from build123d import *

# Parameters (mm, degrees)
BOSS_EXTRUDE1_DEPTH      = 32
CUT_EXTRUDE5_DEPTH       = 3.999999672
LPATTERN1_COUNT          = 5
LPATTERN1_PITCH          = 7
LPATTERN2_COUNT          = 5
LPATTERN2_PITCH          = 6
SKETCH12_W               = 8
SKETCH12_H               = 4
CUT_EXTRUDE7_DEPTH       = 12
CUT_EXTRUDE8_DEPTH       = 17
CUT_EXTRUDE8_DEPTH_BACK  = 4
SKETCH11_W               = 8
SKETCH11_H               = 31.059426665
CUT_EXTRUDE10_DEPTH      = 17
CUT_EXTRUDE10_DEPTH_BACK = 4
SKETCH13_W               = 10.75
SKETCH13_H               = 28.869342983
SKETCH13_W_2             = 7.056880225
SKETCH13_H_2             = 29.936318605
F_4_0MM_DOWEL_HOLE1_D    = 4


with BuildPart() as part:
    # Sketch1 → Boss-Extrude1 (new, symmetric)
    with BuildSketch(Plane.XY):
        Polygon((-23.75, 31.999999672), (23.75, 31.999999672), (23.75, 8), (29, 8), (29, 4), (21, 4), (21, 18), (18.25, 18), (18.25, 28), (-18.25, 28), (-18.25, 18), (-21, 18), (-21, 4), (-29, 4), (-29, 8), (-23.75, 8), align=None)
    extrude(amount=BOSS_EXTRUDE1_DEPTH, both=True)

    # Sketch8 → Cut-Extrude5 (cut)
    with BuildSketch(Plane(origin=(0, 31.999999672, 0), x_dir=(1, 0, 0), z_dir=(0, 1, 0))):
        with BuildLine():
            Line((11.25, -2.8), (-11.25, -2.8))
            ThreePointArc((-11.25, -2.8), (-11.957106781, -2.507106781), (-12.25, -1.8))
            Line((-12.25, -1.8), (-12.25, -1))
            ThreePointArc((-12.25, -1), (-11.957106781, -0.292893219), (-11.25, 0))
            Line((-11.25, 0), (11.25, 0))
            ThreePointArc((11.25, 0), (11.957106781, -0.292893219), (12.25, -1))
            Line((12.25, -1), (12.25, -1.8))
            ThreePointArc((12.25, -1.8), (11.957106781, -2.507106781), (11.25, -2.8))
        make_face()
    cut_extrude5 = extrude(amount=-CUT_EXTRUDE5_DEPTH, mode=Mode.SUBTRACT)

    # LPattern1: Cut-Extrude5 ×5
    with Locations(*[(0, 0, -i * LPATTERN1_PITCH) for i in range(1, LPATTERN1_COUNT)]):
        add(cut_extrude5, mode=Mode.SUBTRACT)

    # LPattern2: Cut-Extrude5 ×5
    with Locations(*[(0, 0, i * LPATTERN2_PITCH) for i in range(1, LPATTERN2_COUNT)]):
        add(cut_extrude5, mode=Mode.SUBTRACT)

    # Sketch12 → Cut-Extrude7 (cut)
    with BuildSketch(Plane(origin=(0, 0, -32), x_dir=(-1, 0, 0), z_dir=(0, 0, -1))):
        with Locations((25, 6)):
            Rectangle(SKETCH12_W, SKETCH12_H)
        with Locations((-25, 6)):
            Rectangle(SKETCH12_W, SKETCH12_H)
    cut_extrude7 = extrude(amount=-CUT_EXTRUDE7_DEPTH, mode=Mode.SUBTRACT)

    # Mirror1: Cut-Extrude7 across plane
    add(cut_extrude7.mirror(Plane.XY), mode=Mode.SUBTRACT)

    # Sketch11 → Cut-Extrude8 (cut, two sides: drawn at the far end of the back side and taken through both)
    with BuildSketch(Plane(origin=(0, 0, -15), x_dir=(-1, 0, 0), z_dir=(0, 0, -1)).offset(-CUT_EXTRUDE8_DEPTH_BACK)):
        with Locations((25, 23.529713333)):
            Rectangle(SKETCH11_W, SKETCH11_H)
        with Locations((-25, 23.529713333)):
            Rectangle(SKETCH11_W, SKETCH11_H)
    extrude(amount=CUT_EXTRUDE8_DEPTH + CUT_EXTRUDE8_DEPTH_BACK, mode=Mode.SUBTRACT)

    # Sketch13 → Cut-Extrude10 (cut, two sides: drawn at the far end of the back side and taken through both)
    with BuildSketch(Plane.XY.offset(15).offset(-CUT_EXTRUDE10_DEPTH_BACK)):
        with Locations((26.375, 22.434671492)):
            Rectangle(SKETCH13_W, SKETCH13_H)
        with Locations((-24.528440113, 22.968159303)):
            Rectangle(SKETCH13_W_2, SKETCH13_H_2)
    extrude(amount=CUT_EXTRUDE10_DEPTH + CUT_EXTRUDE10_DEPTH_BACK, mode=Mode.SUBTRACT)

    # Ø4.0mm Dowel Hole1 (through all)
    with Locations(Plane(origin=(0, 8, 0), x_dir=(1, 0, 0), z_dir=(0, 1, 0))):
        with Locations((25, -15), (25, 15), (-25, 15), (-25, -15)):
            Hole(F_4_0MM_DOWEL_HOLE1_D / 2)


solid = part.part
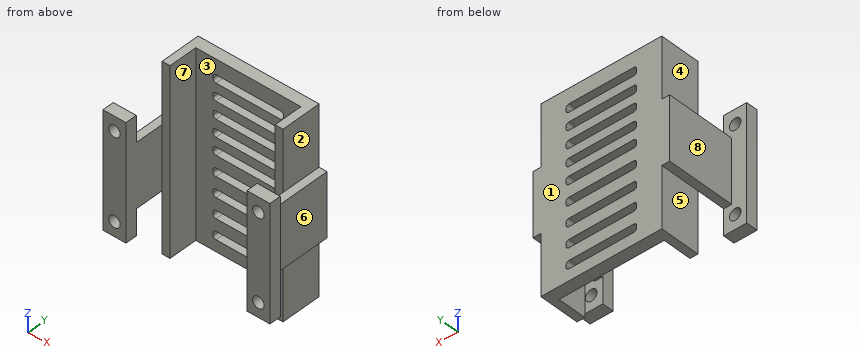
Build history of the part. All positions in model axes, mm. Face numbers are marked on the shaded views. A direction names the side the tool comes from. Coordinates: 2 decimals unless noted, no trailing zeros. Order: outer loops, then holes, each group sorted by start corner. A loop starts at its lowest first (then second) coordinate and runs counter-clockwise, first axis right, second up. Notation, with made-up numbers: (55.5, 4) - (63.5, 4) arc R22 cw to (63.5, 21) - close; hole circle Ø3 at (-23, 80.5). An arc over 180 degrees is marked (long way). Write item = value, one per line. Start each with the question number.
1) Saw through at C-C on y = 10.25. Write the cut outline in (x, z), then the cut area to 3 significant figures.
2) 3-axis set-ups, long thin cutter, end or side, ignore diameter. For the marked faces 4, 5, 6, 7 and 8: which of +Z, -Z, +X, -X, +Y, -Y reach the whole face in a straight line?
3) Wall check: line 1 along X through (y, z) = (6.65, -15); line 2 along Z through (x, y) = (-25, 6.05); line 3 along X through (y, z) = (22.5, -23.5). Give the ranges that are in metal, low to high. Write a range as from..to.
4) Two-plate mould, pull along X, no slides. Class the marked faces 1, 2 and 3: pulls with the +X half, pulls with the -X half, needs draft (parallel to the pull), parting line crosses it, or undercut.
5) Saw through at A-A on z = -15. Write the cut outline in (x, y).
6) Saw through at B-B on x = 25. Write the cut outline in (y, z), then the cut area to 3 significant figures.
7) Saw through at D-D on z = -8. Write the cut outline in (x, y), then the cut area to 3 significant figures.
8) Flat gauge pins, fed straight in: pin 1 Ø4.5 at (x, y) = (27, 5) entering from -Z; pin 2 Ø0.9 at (y, z) = (30, 13.5) entering from -X; pin 3 Ø3 at (y, z) = (21, -3.5) entering from -X; pin 4 Ø3 at (x, z) = (-25, 15) entering from +Y. Where does each tip first touch, or does it go through?
From the geometry:
q1.outline = (-23.75, -11) - (-21, -11) - (-21, 11) - (-23.75, 11) - close; (21, -11) - (23.75, -11) - (23.75, 11) - (21, 11) - close
q1.area = 121 mm^2
q2.face_4 = +Z, -X, +Y
q2.face_5 = -Z, -X, +Y
q2.face_6 = +Z, -Z, +X, +Y
q2.face_7 = +Z, -Z, -Y
q2.face_8 = +Z, -Z, -X, +Y
q3.line_1 = -29..-27, -23..-21, 21..23, 27..29
q3.line_2 = -20..-17, -13..13, 17..20
q3.line_3 = -21..-18.25, 18.25..21
q4.face_1 = needs draft
q4.face_2 = pulls with the +X half
q4.face_3 = undercut
q5.outline = (-29, 4) - (-27, 4) - (-27, 8) - (-29, 8) - close; (-23, 4) - (-21, 4) - (-21, 8) - (-23, 8) - close; (-21, 18) - (-18.25, 18) - (-18.25, 28) - (18.25, 28) - (18.25, 18) - (21, 18) - (21, 32) - (-21, 32) - close; (21, 4) - (23, 4) - (23, 8) - (21, 8) - close; (27, 4) - (29, 4) - (29, 8) - (27, 8) - close
q6.outline = (4, -20) - (8, -20) - (8, -17) - (4, -17) - close; (4, -13) - (8, -13) - (8, 13) - (4, 13) - close; (4, 17) - (8, 17) - (8, 20) - (4, 20) - close
q6.area = 128 mm^2
q7.outline = (-29, 4) - (-21, 4) - (-21, 18) - (-18.25, 18) - (-18.25, 28) - (18.25, 28) - (18.25, 18) - (21, 18) - (21, 4) - (29, 4) - (29, 8) - (23.75, 8) - (23.75, 32) - (-23.75, 32) - (-23.75, 8) - (-29, 8) - close
q7.area = 419 mm^2
q8.pin_1 = -20
q8.pin_2 = -21
q8.pin_3 = -23.75
q8.pin_4 = through
